```python
from build123d import *

# Parameters (mm, degrees)
F0_W     = 19.999999
F0_H     = 33
F0_W_2   = 15
F0_H_2   = 45
F1_DEPTH = 9


with BuildPart() as f1:
    # F0 (on Front) → F1 (new body)
    with BuildSketch(Plane.XZ):
        with BuildLine():
            Line((80.58994, 134.787209), (-99.41006, 134.787209))
            ThreePointArc((-99.41006, 134.787209), (-113.552195, 128.929344), (-119.41006, 114.787209))
            Line((-119.41006, 114.787209), (-119.41006, 109.787209))
            Line((-119.41006, 109.787209), (-111.91006, 109.787209))
            ThreePointArc((-111.91006, 109.787209), (-110.41006, 111.287209), (-108.91006, 109.787209))
            ThreePointArc((-108.91006, 109.787209), (-109.349399, 108.726549), (-110.41006, 108.287209))
            Line((-110.41006, 108.287209), (-110.41006, 94.787209))
            Line((-110.41006, 94.787209), (-90.41006, 94.787209))
            Line((-90.41006, 94.787209), (-90.41006, 104.787209))
            ThreePointArc((-90.41006, 104.787209), (-88.945593, 108.322743), (-85.41006, 109.787209))
            Line((-85.41006, 109.787209), (66.589941, 109.787209))
            ThreePointArc((66.589941, 109.787209), (70.125475, 108.322743), (71.589941, 104.787209))
            Line((71.589941, 104.787209), (71.589941, 84.287209))
            Line((71.589941, 84.287209), (91.58994, 84.287209))
            Line((91.58994, 84.287209), (91.58994, 108.287209))
            ThreePointArc((91.58994, 108.287209), (90.52928, 110.847869), (93.08994, 109.787209))
            Line((93.08994, 109.787209), (100.58994, 109.787209))
            Line((100.58994, 109.787209), (100.58994, 114.787209))
            ThreePointArc((100.58994, 114.787209), (94.732076, 128.929344), (80.58994, 134.787209))
        make_face()
        with BuildLine():
            Line((91.58994, -15.212791), (91.58994, 51.287209))
            Line((91.58994, 51.287209), (71.589941, 51.287209))
            Line((71.589941, 51.287209), (71.589941, 19.787209))
            ThreePointArc((71.589941, 19.787209), (70.125475, 16.251675), (66.589941, 14.787209))
            Line((66.589941, 14.787209), (-9.410059, 14.787209))
            Line((-9.410059, 14.787209), (-9.41006, -5.212791))
            Line((-9.41006, -5.212791), (61.589941, -5.212791))
            ThreePointArc((61.589941, -5.212791), (65.125475, -6.677257), (66.589941, -10.212791))
            Line((66.589941, -10.212791), (66.58994, -35.874643))
            Line((66.58994, -35.874643), (66.589941, -115.212791))
            ThreePointArc((66.589941, -115.212791), (65.125475, -118.748325), (61.589941, -120.212791))
            Line((61.589941, -120.212791), (-85.41006, -120.212791))
            ThreePointArc((-85.41006, -120.212791), (-88.945593, -118.748325), (-90.41006, -115.212791))
            Line((-90.41006, -115.212791), (-90.41006, -110.212791))
            Line((-90.41006, -110.212791), (-110.41006, -110.212791))
            Line((-110.41006, -110.212791), (-110.41006, -118.712791))
            ThreePointArc((-110.41006, -118.712791), (-109.349399, -119.152131), (-108.91006, -120.212791))
            ThreePointArc((-108.91006, -120.212791), (-110.41006, -121.712791), (-111.91006, -120.212791))
            Line((-111.91006, -120.212791), (-119.41006, -120.212791))
            Line((-119.41006, -120.212791), (-119.41006, -125.212791))
            ThreePointArc((-119.41006, -125.212791), (-113.552195, -139.354927), (-99.41006, -145.212791))
            Line((-99.41006, -145.212791), (80.58994, -145.212791))
            ThreePointArc((80.58994, -145.212791), (94.732076, -139.354927), (100.58994, -125.212791))
            Line((100.58994, -125.212791), (100.58994, -120.212791))
            Line((100.58994, -120.212791), (93.08994, -120.212791))
            ThreePointArc((93.08994, -120.212791), (90.52928, -121.273451), (91.58994, -118.712791))
            Line((91.58994, -118.712791), (91.58994, -110.212791))
            Line((91.58994, -110.212791), (91.58994, -60.212791))
            Line((91.58994, -60.212791), (76.58994, -60.212791))
            Line((76.58994, -60.212791), (76.58994, -15.212791))
            Line((76.58994, -15.212791), (91.58994, -15.212791))
        make_face()
        with Locations((81.58994, 67.787209)):
            Rectangle(F0_W, F0_H)
        with Locations((84.08994, -37.712791)):
            Rectangle(F0_W_2, F0_H_2)
    extrude(amount=-F1_DEPTH)


solid = f1.part
```
Can you work these out from the model? Positions are in its coordinate system, mm. A direction names the side the tool comes from. Round coordinates to 2 decimals unless told otherwise and drop trailing zeros. Loops run counter-clockwise (first coordinate to the right, second up) from the corner with the lowest first, then second, coordinate; pieces in that order, holes last. Notation, with made-up numbers: M 4,55 L 24,55 A6 cw 24,61 Z; hole C 43,-33 d3. An arc over 180 degrees is marked long. Write item = value, one per line. Start each with the question number.
(1) Suppose I cut it at A-A on x = 57. Write out the boundary of the cut face in (y, z).
(2) I need wall thicknesses on line 1 along Z through (x, y) = (10.5, 6.25); line 2 along Z through (x, y) = (-60, 2.5); line 3 along X through (y, z) = (1, 96). Which ranges of each line are inside material? Lowest first, please.
(3) Suppose I cut it at C-C on z = 67. Write out the boundary of the cut face in (x, y).
(4) Which directions (+Z, -Z, +X, -X, +Y, -Y) give clear straight access to the entire face, cutting with the end or side of a thin tool? Please do faces 1 (the face through (91.59, 4, 96)), 2 (the face through (-116, 4, 109.787)), 3 (the face through (-10, 4, 109.787)).
(5) If we mould it in two halves opening along Z, with no side actions, what happens to faces 4 (the face through (29, 4, 14.787)), 5 (the face through (71.59, 4, 68)), 6 (the face through (15, 9, -5)), 7 (the face through (-11, 4, -145.213))? For each: released by +Z, released by -Z, zero draft, split by the parting line, or undercut.
(6) Suppose I cut it at B-B on x = -29. Write out the boundary of the cut face in (y, z), plus the area to 3 significant figures.
(7) Suppose I cut it at D-D on z = 7.5. Write out the boundary of the cut face in (x, y).
(8) I'm going to push flat-ended pins straight in: P1, Ø5, axis at y = 6, z = 32.5, coming from the +X side; P2, Ø4.5, axis at y = 6.5, z = 98, coming from the -X side. Where does each tip first touch, or does it pass through?
Answer block:
q1.outline = M 0,-145.21 L 9,-145.21 L 9,-120.21 L 0,-120.21 Z; M 0,-5.21 L 9,-5.21 L 9,14.79 L 0,14.79 Z; M 0,109.79 L 9,109.79 L 9,134.79 L 0,134.79 Z
q2.line_1 = -145.21 to -120.21, -5.21 to 14.79, 109.79 to 134.79
q2.line_2 = -145.21 to -120.21, 109.79 to 134.79
q2.line_3 = -110.41 to -90.41, 71.59 to 91.59
q3.outline = M 71.59,0 L 91.59,0 L 91.59,9 L 71.59,9 Z
q4.face_1 = +X, +Y, -Y
q4.face_2 = -X, +Y, -Y
q4.face_3 = +Y, -Y
q5.face_4 = undercut
q5.face_5 = undercut
q5.face_6 = zero draft
q5.face_7 = released by -Z
q6.outline = M 0,-145.21 L 9,-145.21 L 9,-120.21 L 0,-120.21 Z; M 0,109.79 L 9,109.79 L 9,134.79 L 0,134.79 Z
q6.area = 450 mm²
q7.outline = M -9.41,0 L 91.59,0 L 91.59,9 L -9.41,9 Z
q8.P1 = 91.59
q8.P2 = -110.41
